```python
from build123d import *

# Parameters (mm, degrees)
SKETCH1_W               = 101.6
SKETCH1_H               = 50.8
BOSS_EXTRUDE1_DEPTH     = 6.35
CHAMFER1_SIZE           = 3.175
CHAMFER1_SIZE2          = 25.858299909
CHAMFER2_SIZE           = 3.175
CHAMFER2_SIZE_2         = 25.858299909
CHAMFER3_SIZE           = 3.175
CHAMFER3_SIZE2          = 25.858299909
CHAMFER4_SIZE           = 3.175
CHAMFER4_SIZE_2         = 25.858299909
CUT_EXTRUDE1_DEPTH      = 76.2
CUT_EXTRUDE1_DEPTH_BACK = 25.4


with BuildPart() as part:
    # Sketch1 → Boss-Extrude1 (new body)
    with BuildSketch(Plane(origin=(0, 0, 0), x_dir=(0, 0, -1), z_dir=(1, 0, 0))):
        with Locations((50.8, 25.4)):
            Rectangle(SKETCH1_W, SKETCH1_H)
        Polygon((0, 76.2), (101.6, 50.8), (0, 50.8), align=None)
        Polygon((0, 0), (0, -25.4), (101.6, 0), align=None)
    extrude(amount=BOSS_EXTRUDE1_DEPTH)

    # Chamfer1
    chamfer1_edges = [part.edges().sort_by_distance(p)[0] for p in [
        (0, 63.5, -50.8),
    ]]
    chamfer1_side = [part.faces().sort_by_distance(p)[0] for p in [
        (3.175, 63.5, -50.8),
    ]]
    chamfer(chamfer1_edges, length=CHAMFER1_SIZE, length2=CHAMFER1_SIZE2, reference=chamfer1_side[0])

    # Chamfer2
    # the kernel refuses this chamfer: 25.858299909, 3.175 mm, written as the material it takes off along each edge
    with BuildSketch(Plane(origin=(6.35, 92.501557672, 65.20623069), x_dir=(-0.954887306003921, 0.28810166968922074, -0.07202541742230516), z_dir=(0, -0.24253562503633294, -0.970142500145332))) as chamfer2_piece_1:
        Polygon((CHAMFER2_SIZE * 0.954887306004, -CHAMFER2_SIZE * 0.296968403761), (-CHAMFER2_SIZE_2 * 0.296968403759, -CHAMFER2_SIZE_2 * 0.954887305997), (0, 0), align=None)
    extrude(amount=239.152971182, mode=Mode.SUBTRACT)

    # Chamfer3
    chamfer3_edges = [part.edges().sort_by_distance(p)[0] for p in [
        (0, -12.7, -50.8),
    ]]
    chamfer3_side = [part.faces().sort_by_distance(p)[0] for p in [
        (3.175, -12.7, -50.8),
    ]]
    chamfer(chamfer3_edges, length=CHAMFER3_SIZE, length2=CHAMFER3_SIZE2, reference=chamfer3_side[0])

    # Chamfer4
    # the kernel refuses this chamfer: 25.858299909, 3.175 mm, written as the material it takes off along each edge
    with BuildSketch(Plane(origin=(6.35, -41.701557672, 65.20623069), x_dir=(-0.9548873060039216, -0.2881016696892189, -0.07202541742230473), z_dir=(0, 0.24253562503633297, -0.9701425001453319))) as chamfer4_piece_1:
        Polygon((CHAMFER4_SIZE * 0.954887306004, CHAMFER4_SIZE * 0.296968403761), (-CHAMFER4_SIZE_2 * 0.296968403759, CHAMFER4_SIZE_2 * 0.954887305997), (0, 0), align=None)
    extrude(amount=239.152971182, mode=Mode.SUBTRACT)

    # Sketch2 → Cut-Extrude1 (cut, two sides: drawn at the far end of the back side and taken through both)
    with BuildSketch(Plane(origin=(0, 0, 0), x_dir=(1, 0, 0), z_dir=(0, 1, 0)).offset(-CUT_EXTRUDE1_DEPTH_BACK)):
        with BuildLine():
            Line((3.175, -34.036), (-2.377874902, -0.404533862))
            ThreePointArc((-2.377874902, -0.404533862), (3.986335677, 0.041142906), (10.322125098, -0.706905547))
            Line((10.322125098, -0.706905547), (3.175, -34.036))
        make_face()
    extrude(amount=CUT_EXTRUDE1_DEPTH + CUT_EXTRUDE1_DEPTH_BACK, mode=Mode.SUBTRACT)


solid = part.part
```
Could you check a few things on this model? Use its own coordinates, in mm. Round coordinates to 2 decimals unless told otherwise and drop trailing zeros. Write each loop counter-clockwise with the first axis right and the second up, starting at its lowest first coordinate (ties: lowest second). Pieces come first, ordered by that corner, then holes. Notation, with made-up numbers: M 38,-17.75 L 59,-17.75 A16 ccw 59,-2.75 Z; hole C 39,14.5 d4. An arc over 180 degrees is marked long. Answer in a Markdown table with one row per item. Add a question column.
Q1. If I drill on line 1 (Z direction, x = 2, y = 24.5); line 2 (X direction, y = 13, z = -91); line 3 (X direction, y = 30.5, z = -96), over which ranges is the centre line in solid material (lowest first)? Write a range as from..to.
Q2. Will these pins go through, and if not, where does the flat tip stop? pin 1 Ø10 at (y, z) = (59.5, -16.5) entering from +X; pin 2 Ø3 at (y, z) = (35.5, -62.5) entering from -X; pin 3 Ø1.5 at (y, z) = (16.5, -89.5) entering from +X.
Q3. Imagine slicing it at B-B (y = 53.5). Please give me the cut outline in (x, z) (3 decimals).
Q4. Imagine slicing it at C-C (z = -13.5). Please give me the cut outline in (x, y) (3 decimals).
Q5. Imagine slicing it at A-A (z = -25). Please give me the cut outline in (x, y) (3 decimals).
Q6. Imagine slicing it at D-D (y = -17). Please give me the cut outline in (x, z) (3 decimals), then the cut area to 3 significant figures.
Values:
| question | item | result |
|---|---|---|
| 1 | line 1 | -101.6..-0.03 |
| 1 | line 2 | 1.31..5.04 |
| 1 | line 3 | 0.59..5.76 |
| 2 | pin 1 | x = 5.29 |
| 2 | pin 2 | x = 0 |
| 2 | pin 3 | x = 5.59 |
| 3 | outline | M 0.471,0 L 3.175,-90.8 L 5.879,0 L 5.035,0 A34.087 cw 1.315,0 Z |
| 4 | outline | M 0,4.629 L 3.175,-22.025 L 6.35,4.629 L 6.35,46.171 L 3.175,72.825 L 0,46.171 Z |
| 5 | outline | M 0,7.504 L 3.175,-19.15 L 6.35,7.504 L 6.35,43.296 L 3.175,69.95 L 0,43.296 Z |
| 6 | outline | M 2.175,-0.036 L 3.175,-33.6 L 4.175,-0.036 A34.087 cw Z |
| 6 | area | 33.5 mm^2 |
